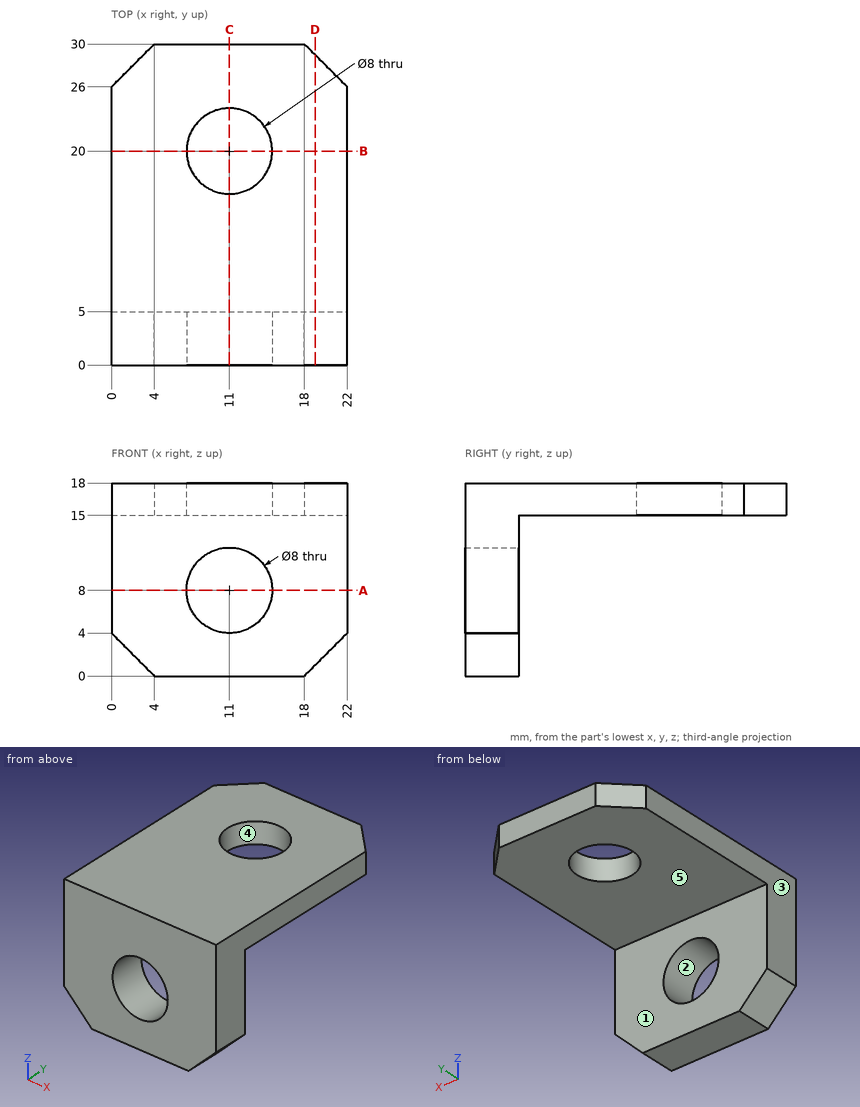
Here's the drawing with two shaded views (mm, measured from the low corner). I have some questions. A direction names the side the tool comes from. Coordinates: 2 decimals unless noted, no trailing zeros. Write each loop counter-clockwise with the first axis right and the second up, starting at its lowest first coordinate (ties: lowest second). Pieces come first, ordered by that corner, then holes. Notation, with made-up numbers: (42.25, 74) - (91.25, 74) arc R31 cw to (91.25, 104) - close; hole circle Ø10 at (-17, -9). An arc over 180 degrees is marked (long way). Return JSON: item names as keys, results as strings.
Q1. If we section it at C-C (x = 11): Please give me the cut outline in (y, z), then the cut area to 3 significant figures.
Computed values:
{"outline": "(0, 0) - (5, 0) - (5, 4) - (0, 4) - close; (0, 12) - (5, 12) - (5, 15) - (16, 15) - (16, 18) - (0, 18) - close; (24, 15) - (30, 15) - (30, 18) - (24, 18) - close", "area": "101 mm2"}
Q2. On a 3-axis mill with a long thin cutter (end or side, diameter ignored), from which of +Z, -Z, +X, -X, +Y, -Y can I reach the whole of each face in a straight line? I mean the marked faces 1 and 2. Say none if no direction works.
Computed values:
{"face 1": "-Z, +X, -X, +Y", "face 2": "+Y, -Y"}
Q3. Please list where these lines run through material, in increasing order: L1, parallel to X at y = 1.3, z = 8; L2, parallel to Y at x = 11, z = 16.15; L3, parallel to Y at x = 2.75, z = 8.75. Write a range as from..to.
Computed values:
{"L1": "x = 0..7, 15..22", "L2": "y = 0..16, 24..30", "L3": "y = 0..5"}
Q4. If we section it at D-D (x = 19): Please give me the cut outline in (y, z), then the cut area to 3 significant figures.
Computed values:
{"outline": "(0, 1) - (5, 1) - (5, 15) - (29, 15) - (29, 18) - (0, 18) - close", "area": "157 mm2"}
Q5. I'm going to push a flat-ended pin straight in: pin 1 Ø3 at (x, y) = (6, 23) entering from -Z. Where does the tip first touch, or does it pass through?
Computed values:
{"pin 1": "stops at z = 15"}
Q6. If we section it at B-B (y = 20): Please give me the cut outline in (x, z).
Computed values:
{"outline": "(0, 15) - (7, 15) - (7, 18) - (0, 18) - close; (15, 15) - (22, 15) - (22, 18) - (15, 18) - close"}
Q7. Thinking about a two-plate mould opening in X: for the marked faces 3, 4 and 5, which applies, +X half, -X half, draft (parallel to the pull), parting line (faces both ways), or undercut?
Computed values:
{"face 3": "-X half", "face 4": "undercut", "face 5": "draft"}
Q8. If we section it at A-A (z = 8): Please give me the cut outline in (x, y).
Computed values:
{"outline": "(0, 0) - (7, 0) - (7, 5) - (0, 5) - close; (15, 0) - (22, 0) - (22, 5) - (15, 5) - close"}
